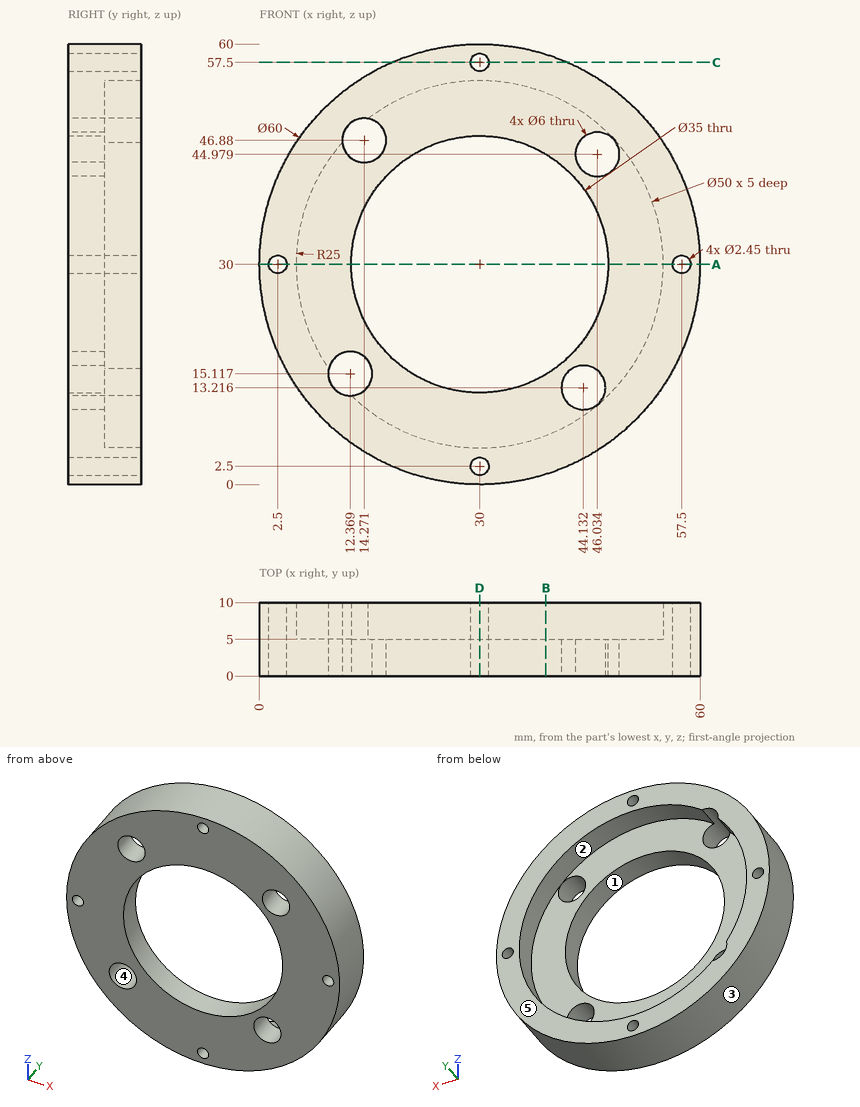
Verification items for this drawing (mm, ordinates from the low corner). A direction names the side the tool comes from. Give positions to 0.01 mm unless a question says otherwise; leave off trailing zeros. Loops run counter-clockwise (first coordinate to the right, second up) from the corner with the lowest first, then second, coordinate; pieces in that order, holes last.
(1) Depth check by flat-ended pin: pin 1 Ø2 at (y, z) = (2.5, 43.5) entering from -X; pin 2 Ø7 at (x, z) = (14.27, 46.88) entering from -Y; pin 3 Ø1.5 at (y, z) = (8, 22.5) entering from -X; pin 4 Ø5 at (x, y) = (47.5, 4.5) entering from +Z. Enter the tip coordinate at first touch or a pass-through.
From the geometry:
pin 1: stops at x = 2.73
pin 2: stops at y = 0
pin 3: stops at x = 0.77
pin 4: stops at z = 55.98
(2) Section check A-A on z = 30. Record the cut outline in (x, y) (1 decimal).
From the geometry:
outline: (0, 0) - (1.3, 0) - (1.3, 10) - (0, 10) - close; (3.7, 0) - (12.5, 0) - (12.5, 5) - (5, 5) - (5, 10) - (3.7, 10) - close; (47.5, 0) - (56.3, 0) - (56.3, 10) - (55, 10) - (55, 5) - (47.5, 5) - close; (58.7, 0) - (60, 0) - (60, 10) - (58.7, 10) - close
(3) Section check B-B on x = 39. Record the cut outline in (y, z), then the cut area to 3 significant figures.
From the geometry:
outline: (0, 1.38) - (10, 1.38) - (10, 6.68) - (5, 6.68) - (5, 14.99) - (0, 14.99) - close; (0, 45.01) - (5, 45.01) - (5, 53.32) - (10, 53.32) - (10, 58.62) - (0, 58.62) - close
area: 189 mm2
(4) Release check for a two-part mould opening along X. For the marked faces 3, 4 and 5 record: released by +X, released by -X, zero draft, split by the parting line, or undercut.
From the geometry:
face 3: split by the parting line
face 4: undercut
face 5: zero draft
(5) Section check D-D on x = 30. Record the cut outline in (y, z) (1 decimal), then the cut area to 3 significant figures.
From the geometry:
outline: (0, 0) - (10, 0) - (10, 1.3) - (0, 1.3) - close; (0, 3.7) - (10, 3.7) - (10, 5) - (5, 5) - (5, 12.5) - (0, 12.5) - close; (0, 47.5) - (5, 47.5) - (5, 55) - (10, 55) - (10, 56.3) - (0, 56.3) - close; (0, 58.7) - (10, 58.7) - (10, 60) - (0, 60) - close
area: 126 mm2
(6) Thickness scan on L1, parallel to Z at x = 30, y = 6 (1 decimal); L2, parallel to X at y = 6.5, z = 12; L3, parallel to Z at x = 37.5, y = 6.5. Record the ranges inside material, lowest first.
From the geometry:
L1: z = 0 to 1.3, 3.7 to 5, 55 to 56.3, 58.7 to 60
L2: x = 6 to 12.65, 47.35 to 54
L3: z = 0.95 to 6.15, 53.85 to 59.05
(7) Section check C-C on z = 57.5. Record the cut outline in (x, y) (1 decimal), then the cut area to 3 significant figures.
From the geometry:
outline: (18, 0) - (28.8, 0) - (28.8, 10) - (18, 10) - close; (31.2, 0) - (42, 0) - (42, 10) - (31.2, 10) - close
area: 215 mm2
(8) Set-up check for the marked faces 1 and 2: record each of +Z, -Z, +X, -X, +Y, -Y from which the full face is reachable in a straight line by a thin tool's end or side.
From the geometry:
face 1: +Y, -Y
face 2: +Y
